The model under review builds one solid part; all positions refer to its coordinate system, in mm. Give positions to 0.01 mm unless a question says otherwise; leave off trailing zeros. Order: outer loops, then holes, each group sorted by start corner. A loop starts at its lowest first (then second) coordinate and runs counter-clockwise, first axis right, second up. Notation, with made-up numbers: (36, 12.5) - (55, 12.5) arc R26 ccw to (55, 49.5) - close; hole circle Ø11 at (35, 34). An arc over 180 degrees is marked (long way). Use CSV: the item, a comma, the result in double quotes. Start each with the question number.
1. Take a section at C-C, the plane z = 2. State the section outline as (x, y) points.
2. Take a section at B-B, the plane z = -10.5. State the section outline as (x, y) points, then the cut area to 3 significant figures.
3. Take a section at A-A, the plane x = 14. State the section outline as (y, z) points, then the cut area to 3 significant figures.
4. For pin 1 (3 mm diameter, centred on x = 23, y = 4, fed in from +Z); pin 2 (0.8 mm diameter, centred on y = 4, z = 0.5, fed in from +X); pin 3 (1.8 mm diameter, centred on x = -39, y = 3.5, fed in from -Z), all flat-tipped, find the tip position at first contact; note any pin that passes through.
5. To check wall thickness, follow line 1 (Z direction, x = 3.5, y = 5); line 2 (X direction, y = 0.7, z = 2.5); line 3 (X direction, y = 4.2, z = -11). State the ranges of each line that lie inside material, in increasing order. Write a range as [from, to].
6. Take a section at D-D, the plane y = 4.05. Count the separate pieces of the cut face and the enclosed holes in it, then the cut area to 3 significant figures.
Autodesk Inventor part; units mm, degrees
ref_plane "YZ Plane" through (0, 0, 0) normal (1, 0, 0) x (0, 1, 0)
ref_plane "XZ Plane" through (0, 0, 0) normal (0, 1, 0) x (-1, 0, 0)
ref_plane "XY Plane" through (0, 0, 0) normal (0, 0, 1) x (1, 0, 0)
sketch "Sketch1" plane through (0, 0, 0) normal (1, 0, 0) x (0, 1, 0)
  point P0 (0, 0)
sketch "Sketch2" plane through (0, 0, 0) normal (0, 1, 0) x (-1, 0, 0)
  line L0 (0, 0) -> (35, 0)
  line L1 (35, -21) -> (0, -21)
  line L2 (35, -7) -> (41, -7)
  line L3 (41, -7) -> (41, -14)
  line L4 (41, -14) -> (35, -14)
  line L5 (35, 0) -> (35, -7)
  line L6 (35, -14) -> (35, -21)
  line L7 (0, -21) -> (-40, -21)
  line L8 (-40, -21) -> (-40, 0)
  line L9 (-40, 0) -> (0, 0)
  circle A0 centre (-34, -10.5) radius 2.1
  circle A1 centre (-14, -10.5) radius 2.1
  line L10 (0, -7) -> (-6, -7)
  line L11 (-6, -7) -> (-6, -14)
  line L12 (-6, -14) -> (0, -14)
  line L13 (0, -14) -> (0, -7)
  dimension "d0" = 35
  dimension "d1" = 21
  dimension "d2" = 7
  dimension "d3" = 6
  dimension "d4" = 7
  dimension "d5" = 40
  dimension "d8" = 4.2
  dimension "d10" = 4.2
  dimension "d11" = 6
  dimension "d12" = 7
extrude "Extrusion1" add sketch "Sketch2" along normal blind 6
sketch "Sketch3" plane through (0, 6, 0) normal (0, 1, 0) x (1, 0, 0)
  line L0 (0, -1) -> (-35, -1)
  line L1 (-35, 0) -> (40, 0)
  line L2 (-35, -1) -> (-35, 0)
  line L3 (-35, 21) -> (-35, 14)
  line L4 (-35, 21) -> (6, 21)
  line L5 (6, 21) -> (6, 22)
  line L6 (6, 22) -> (-35, 22)
  line L7 (-35, 22) -> (-35, 21)
  line L8 (0, -1) -> (6, -1)
  line L9 (6, -1) -> (6, 0)
  point P0 (0, 0)
  dimension "d15" = 1
  dimension "d17" = 41
  dimension "d18" = 1
  dimension "d21" = 6
extrude "Extrusion2" add sketch "Sketch3" against normal blind 6
sketch "Sketch4" plane through (0, 6, 0) normal (0, 1, 0) x (1, 0, 0)
  line L0 (6, -1) -> (-35, -1)
  line L1 (0, -1) -> (-7, -1)
  line L2 (-7, -1) -> (-7, -7)
  line L3 (-7, -7) -> (0, -7)
  line L4 (0, -7) -> (0, -1)
  line L5 (6, 22) -> (-35, 22)
  line L6 (0, 22) -> (-7, 22)
  line L7 (-7, 22) -> (-7, 28)
  line L8 (-7, 28) -> (0, 28)
  line L9 (0, 28) -> (0, 22)
  point P0 (0, 0)
  dimension "d22" = 7
  dimension "d23" = 6
  dimension "d24" = 7
  dimension "d25" = 6
extrude "Extrusion3" add sketch "Sketch4" against normal blind 6
pattern_linear "Rectangular Pattern1" count 3 spacing 14 along (-1, 0, 0) of "Extrusion3"
properties part number "g_arm_v_1"
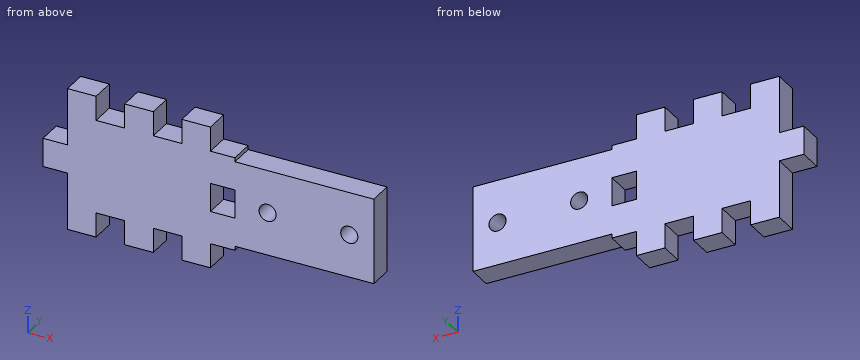
Determined:
1,outline,"(-35, 0) - (-28, 0) - (-28, 6) - (-35, 6) - close; (-21, 0) - (-14, 0) - (-14, 6) - (-21, 6) - close; (-7, 0) - (0, 0) - (0, 6) - (-7, 6) - close"
2,outline,"(-41, 0) - (0, 0) - (0, 6) - (-41, 6) - close; (6, 0) - (11.9, 0) - (11.9, 6) - (6, 6) - close; (16.1, 0) - (31.9, 0) - (31.9, 6) - (16.1, 6) - close; (36.1, 0) - (40, 0) - (40, 6) - (36.1, 6) - close"
2,area,"400 mm²"
3,outline,"(0, -21) - (6, -21) - (6, -12.6) - (0, -12.6) - close; (0, -8.4) - (6, -8.4) - (6, 0) - (0, 0) - close"
3,area,"101 mm²"
4,pin 1,"stops at z = 0"
4,pin 2,"stops at x = 6"
4,pin 3,"stops at z = -14"
5,line 1,"z = [-22, -14], [-7, 1]"
5,line 2,"x = [-35, -28], [-21, -14], [-7, 0]"
5,line 3,"x = [-41, 0], [6, 11.96], [16.04, 31.96], [36.04, 40]"
6,separate pieces,"1"
6,enclosed holes,"3"
6,area,"1,880 mm²"
